Could you check a few things on this model? Use its own coordinates, in mm. Give positions to 0.01 mm unless a question says otherwise; leave off trailing zeros. Order: outer loops, then holes, each group sorted by start corner. A loop starts at its lowest first (then second) coordinate and runs counter-clockwise, first axis right, second up. Notation, with made-up numbers: M -31,82.25 L -6,82.25 A25 cw -6,121.25 Z; hole C 4.25,-26.5 d4. An arc over 180 degrees is marked long. Use a Markdown table: item, result. Add a question column.
Item 1: Suppose I cut it at B-B on x = 6.5. Write out the boundary of the cut face in (y, z), plus the area to 3 significant figures.
Item 2: I'm going to push flat-ended pins straight in: pin 1 Ø1.5 at (x, y) = (35.5, 1) entering from -Z; pin 2 Ø8 at (x, z) = (-6, -59.5) entering from -Y; pin 3 Ø1 at (y, z) = (0.5, -18.5) entering from -X; pin 4 Ø0.9 at (y, z) = (2, -20) entering from +X. Where does each tip first touch, or does it pass through?
Item 3: Suppose I cut it at A-A on z = -62. Write out the boundary of the cut face in (x, y).
Item 4: If I drill on L1, parallel to Z at x = 0, y = 1.5; L2, parallel to X at y = 2.3, z = -77; L3, parallel to Z at x = -20.5, y = 0.3 (3 decimals), over which ranges is the centre line in solid material (lowest first)? Write a range as from..to.
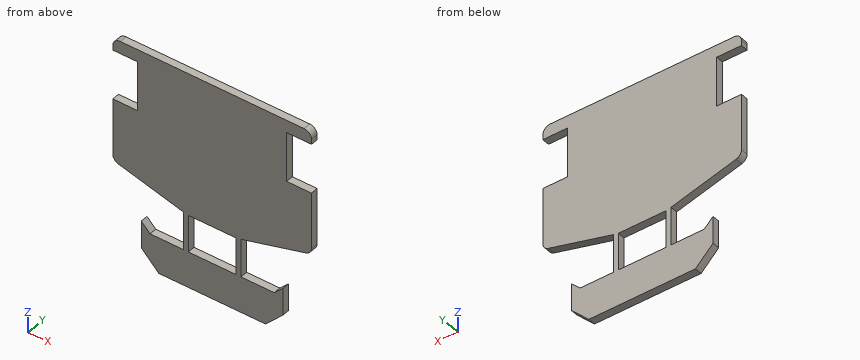
from build123d import *

# Parameters (mm, degrees)
BOSS_EXTRUDE1_DEPTH = 3
BOSS_EXTRUDE2_DEPTH = 3
BOSS_EXTRUDE3_DEPTH = 3


with BuildPart() as part:
    # Sketch1 → Boss-Extrude1 (new body)
    with BuildSketch(Plane(origin=(0, 0, 0), x_dir=(1, 0, 0), z_dir=(0, 1, 0))):
        with BuildLine():
            Line((9.605042507, 58.038475773), (-9.605042507, 58.038475773))
            ThreePointArc((-9.605042507, 58.038475773), (-9.996621084, 58.012810357), (-10.381499643, 57.936253252))
            Line((-10.381499643, 57.936253252), (-37.776457135, 50.595796515))
            ThreePointArc((-37.776457135, 50.595796515), (-39.380060021, 49.524303323), (-40, 47.698019036))
            Line((-40, 47.698019036), (-40, 25))
            Line((-40, 25), (-30, 25))
            Line((-30, 25), (-30, 5))
            Line((-30, 5), (-40, 5))
            Line((-40, 5), (-40, 3))
            ThreePointArc((-40, 3), (-39.121320344, 0.878679656), (-37, 0))
            Line((-37, 0), (37, 0))
            ThreePointArc((37, 0), (39.121320344, 0.878679656), (40, 3))
            Line((40, 3), (40, 5))
            Line((40, 5), (30, 5))
            Line((30, 5), (30, 25))
            Line((30, 25), (40, 25))
            Line((40, 25), (40, 47.698019036))
            ThreePointArc((40, 47.698019036), (39.380060021, 49.524303323), (37.776457135, 50.595796515))
            Line((37.776457135, 50.595796515), (10.381499643, 57.936253252))
            ThreePointArc((10.381499643, 57.936253252), (9.996621084, 58.012810357), (9.605042507, 58.038475773))
        make_face()
    extrude(amount=BOSS_EXTRUDE1_DEPTH)

    # Sketch3 → Boss-Extrude2 (add)
    with BuildSketch(Plane(origin=(0, 3, 0), x_dir=(1, 0, 0), z_dir=(0, 1, 0))):
        Polygon((-11.605042507, 57.608405929), (-9.605042507, 58.038475773), (-9.605042507, 73.038475773), (-11.605042507, 73.038475773), align=None)
        Polygon((9.605042507, 73.038475773), (9.605042507, 58.038475773), (11.605042507, 57.608405929), (11.605042507, 73.038475773), align=None)
    extrude(amount=-BOSS_EXTRUDE2_DEPTH)

    # Sketch4 → Boss-Extrude3 (add)
    with BuildSketch(Plane(origin=(0, 3, 0), x_dir=(1, 0, 0), z_dir=(0, 1, 0))):
        Polygon((0, 73.038475773), (-25, 73.038475773), (-28.535533906, 69.502941867), (-28.535533906, 80.502941867), (-21.464466094, 87.574009679), (21.464466094, 87.574009679), (28.535533906, 80.502941867), (28.535533906, 69.502941867), (25, 73.038475773), align=None)
    extrude(amount=-BOSS_EXTRUDE3_DEPTH)


solid = part.part
Findings below:
| question | item | result |
|---|---|---|
| 1 | outline | M 0,-87.57 L 3,-87.57 L 3,-73.04 L 0,-73.04 Z; M 0,-58.04 L 3,-58.04 L 3,0 L 0,0 Z |
| 1 | area | 218 mm^2 |
| 2 | pin 1 | stops at z = -51.41 |
| 2 | pin 2 | stops at y = 0 |
| 2 | pin 3 | stops at x = -30 |
| 2 | pin 4 | stops at x = 30 |
| 3 | outline | M -11.61,0 L -9.61,0 L -9.61,3 L -11.61,3 Z; M 9.61,0 L 11.61,0 L 11.61,3 L 9.61,3 Z |
| 4 | L1 | z = -87.57..-73.04, -58.04..0 |
| 4 | L2 | x = -28.54..28.54 |
| 4 | L3 | z = -87.574..-73.038, -55.225..0 |
